For this review, use the dimensioned drawing (mm, ordinates from the lowest corner) and the shaded views. Give positions to 0.01 mm unless a question says otherwise; leave off trailing zeros. Write each loop counter-clockwise with the first axis right and the second up, starting at its lowest first coordinate (ties: lowest second). Pieces come first, ordered by that corner, then holes.
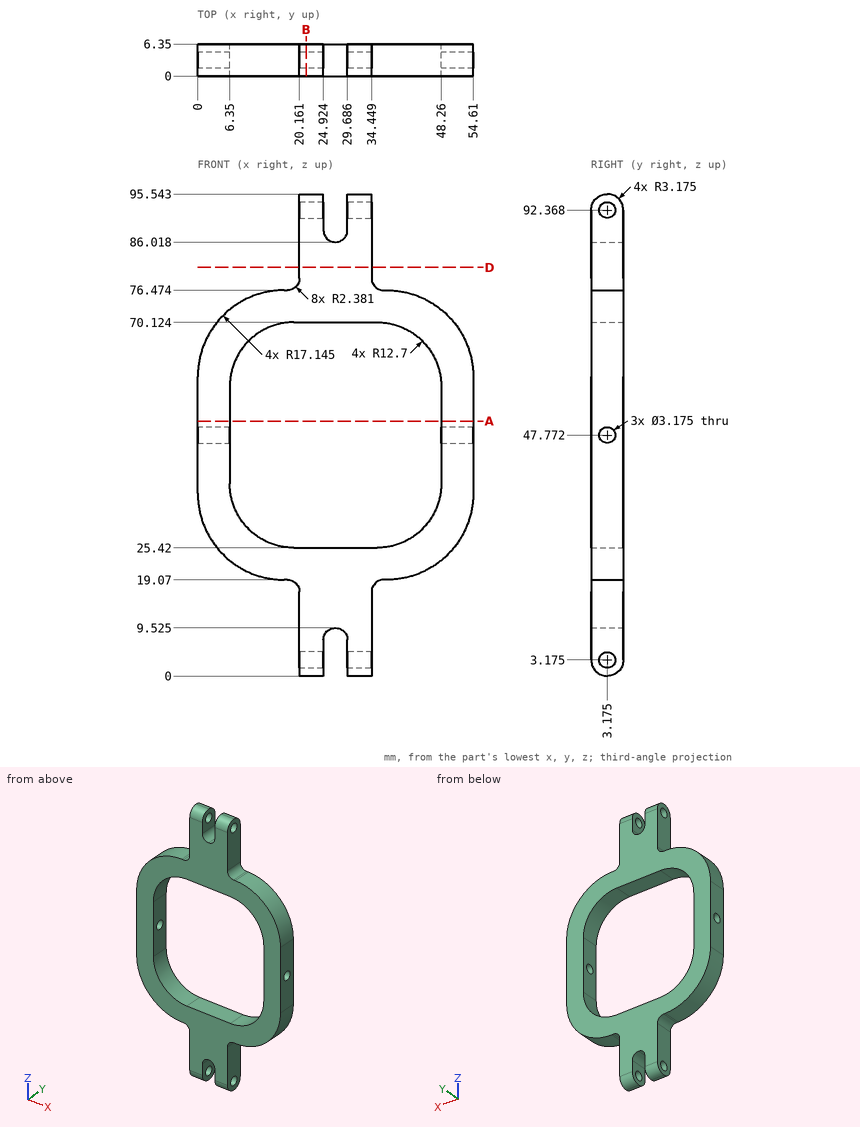
(1) Clearance check with flat-ended pins moving along their axes: pin 1 Ø10 at (x, z) = (16.5, 67.5) entering from -Y; pin 2 Ø1 at (x, y) = (33, 4.5) entering from -Z; pin 3 Ø1 at (x, y) = (37.5, 1.5) entering from -Z; pin 4 Ø1.9 at (x, y) = (27, 3) entering from -Z. State where each tip first meets the part, or that it passes through.
(2) We need section D-D (z = 81). Write out the cut boundary in (x, y).
(3) We need section B-B (x = 21.5). Count the separate pieces of the cut face and the enclosed holes in it, and give its area (3 significant figures).
(4) For L1, parallel to X at y = 2, z = 38.5; L2, parallel to Z at x = 21, y = 1.75 (1 decimal), list the stretches that pass through material, from the lowest coordinate up.
(5) We need section A-A (z = 50.5). Write out the cut boundary in (x, y).
The answers:
1. pin 1: stops at y = 0
1. pin 2: stops at z = 0.11
1. pin 3: stops at z = 19.07
1. pin 4: stops at z = 9.17
2. outline: (20.16, 0) - (34.45, 0) - (34.45, 6.35) - (20.16, 6.35) - close
3. separate pieces: 2
3. enclosed holes: 2
3. area: 298 mm2
4. L1: x = 0 to 6.35, 48.26 to 54.61
4. L2: z = 0.3 to 2.5, 3.9 to 25.4, 70.1 to 91.7, 93.1 to 95.2
5. outline: (0, 0) - (6.35, 0) - (6.35, 6.35) - (0, 6.35) - close; (48.26, 0) - (54.61, 0) - (54.61, 6.35) - (48.26, 6.35) - close
